Answer from the drawing. Dimensions are ordinates in mm from the lowest x, y and z of the part. A direction names the side the tool comes from. Coordinates: 2 decimals unless noted, no trailing zeros. Order: outer loops, then holes, each group sorted by start corner. A loop starts at its lowest first (then second) coordinate and runs counter-clockwise, first axis right, second up. Notation, with made-up numbers: (27.5, 59) -> (47.5, 59) arc R11 ccw to (47.5, 72) -> close; hole circle Ø9 at (77, -31.5). An arc over 180 degrees is marked (long way). Use CSV: the item, a comma, the result in double quotes.
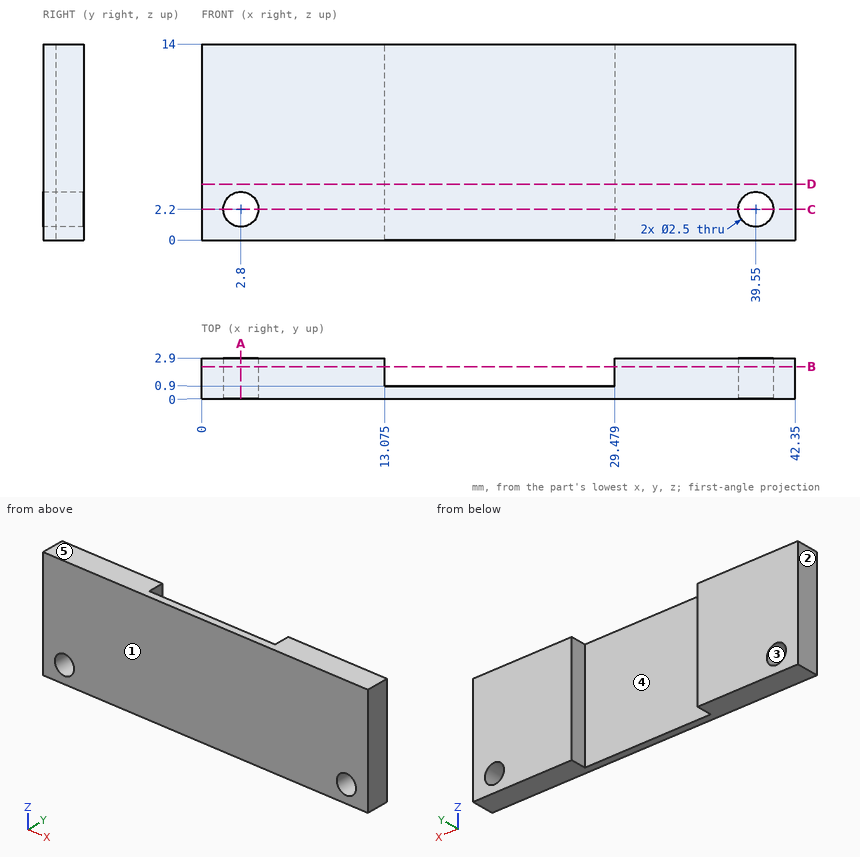
Item 1: Find section A-A, the plane x = 2.8. Give the vertices of the cut face in (y, z).
Return value:
outline,"(0, 0) -> (2.9, 0) -> (2.9, 0.95) -> (0, 0.95) -> close; (0, 3.45) -> (2.9, 3.45) -> (2.9, 14) -> (0, 14) -> close"
Item 2: Find section D-D, the plane z = 4. Give the vertices of the cut face in (x, y) (3 decimals).
Return value:
outline,"(0, 0) -> (42.35, 0) -> (42.35, 2.9) -> (29.479, 2.9) -> (29.479, 0.9) -> (13.075, 0.9) -> (13.075, 2.9) -> (0, 2.9) -> close"
Item 3: Each of these flat-tipped pins is pushed along its axis until it touches: P1, Ø6, axis at x = 24.5, z = 12, coming from the +Y side; P2, Ø0.6, axis at y = 2.5, z = 8.5, coming from the -X side. Where does it stop, or does it pass through?
Return value:
P1,"stops at y = 0.9"
P2,"stops at x = 0"
Item 4: Find section B-B, the plane y = 2.3. Give the vertices of the cut face in (x, z) (3 decimals).
Return value:
outline,"(0, 0) -> (13.075, 0) -> (13.075, 14) -> (0, 14) -> close; (29.479, 0) -> (42.35, 0) -> (42.35, 14) -> (29.479, 14) -> close; hole circle Ø2.5 at (2.8, 2.2); hole circle Ø2.5 at (39.55, 2.2)"
Item 5: A tool of negligible diameter and unlimited length cuts with its end or side. For the marked faces 4 and 5, from which of +Z, -Z, +X, -X, +Y, -Y can it reach the whole face along a straight path? Write none if from no direction.
Return value:
face 4,"+Z, -Z, +Y"
face 5,"+Z, +X, -X, +Y, -Y"
Item 6: Find section C-C, the plane z = 2.2. Give the vertices of the cut face in (x, y) (3 decimals), then the cut area to 3 significant figures.
Return value:
outline,"(0, 0) -> (1.55, 0) -> (1.55, 2.9) -> (0, 2.9) -> close; (4.05, 0) -> (38.3, 0) -> (38.3, 2.9) -> (29.479, 2.9) -> (29.479, 0.9) -> (13.075, 0.9) -> (13.075, 2.9) -> (4.05, 2.9) -> close; (40.8, 0) -> (42.35, 0) -> (42.35, 2.9) -> (40.8, 2.9) -> close"
area,"75.5 mm^2"
Item 7: The mould has two halves that part along X. Classify the marked faces 1, 2 and 3: +X half, -X half, draft (parallel to the pull), parting line (faces both ways), or undercut.
Return value:
face 1,"draft"
face 2,"-X half"
face 3,"undercut"
Item 8: Straight lines are drawn through the part: line 1 along X through (y, z) = (0.6, 2.2); line 2 along X through (y, z) = (1.15, 2.2) (3 decimals); line 3 along X through (y, z) = (2.6, 7.5) (3 decimals). For each, find the intervals that lie inside material, in ascending order.
Return value:
line 1,"x = 0 to 1.55, 4.05 to 38.3, 40.8 to 42.35"
line 2,"x = 0 to 1.55, 4.05 to 13.075, 29.479 to 38.3, 40.8 to 42.35"
line 3,"x = 0 to 13.075, 29.479 to 42.35"
